Here's how the part is built. I have some questions about the finished solid (model axes, mm). Face numbers are marked on the shaded views. Give positions to 0.01 mm unless a question says otherwise; leave off trailing zeros. Order: outer loops, then holes, each group sorted by start corner. A loop starts at its lowest first (then second) coordinate and runs counter-clockwise, first axis right, second up. Notation, with made-up numbers: (-27, 70) - (-13, 70) arc R20 ccw to (-13, 81) - close; hole circle Ø1 at (72, 51.5). An arc over 180 degrees is marked (long way). One line per question, with ' | ' between items.
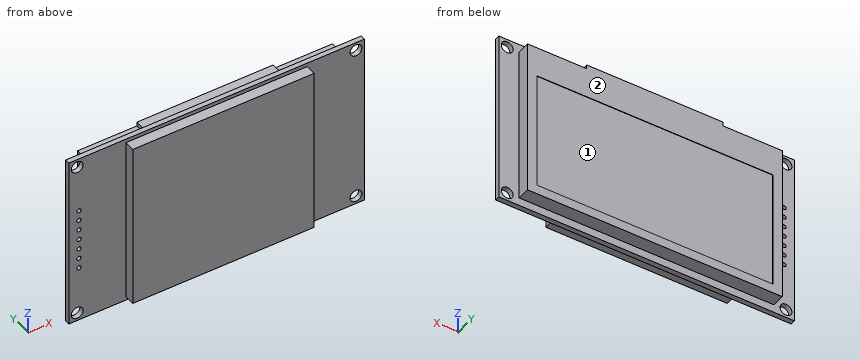
from build123d import *

# Parameters (mm, degrees)
SKETCH1_W           = 72.5
SKETCH1_H           = 43
SKETCH1_R           = 1.45
SKETCH1_R_2         = 0.5
BOSS_EXTRUDE1_DEPTH = 1.2
SKETCH2_W           = 44.5
SKETCH2_H           = 41.146019014
BOSS_EXTRUDE2_DEPTH = 2.6
BOSS_EXTRUDE3_DEPTH = 3.13
SKETCH4_W           = 57.9
SKETCH4_H           = 29.2
CUT_EXTRUDE1_DEPTH  = 0.1


with BuildPart() as part:
    # Sketch1 → Boss-Extrude1 (new body)
    with BuildSketch(Plane(origin=(0, 0, 0), x_dir=(1, 0, 0), z_dir=(0, 1, 0))):
        Rectangle(SKETCH1_W, SKETCH1_H)
        with Locations((-34.2, 19.45)):
            Circle(SKETCH1_R, mode=Mode.SUBTRACT)
        with Locations((-33.75, 7.62)):
            Circle(SKETCH1_R_2, mode=Mode.SUBTRACT)
        with Locations((-33.75, 5.08)):
            Circle(SKETCH1_R_2, mode=Mode.SUBTRACT)
        with Locations((-33.75, 2.54)):
            Circle(SKETCH1_R_2, mode=Mode.SUBTRACT)
        with Locations((-33.75, 0)):
            Circle(SKETCH1_R_2, mode=Mode.SUBTRACT)
        with Locations((-33.75, -2.54)):
            Circle(SKETCH1_R_2, mode=Mode.SUBTRACT)
        with Locations((-33.75, -5.08)):
            Circle(SKETCH1_R_2, mode=Mode.SUBTRACT)
        with Locations((-33.75, -7.62)):
            Circle(SKETCH1_R_2, mode=Mode.SUBTRACT)
        with Locations((-34.2, -19.45)):
            Circle(SKETCH1_R, mode=Mode.SUBTRACT)
        with Locations((34.2, 19.45)):
            Circle(SKETCH1_R, mode=Mode.SUBTRACT)
        with Locations((34.2, -19.45)):
            Circle(SKETCH1_R, mode=Mode.SUBTRACT)
    extrude(amount=-BOSS_EXTRUDE1_DEPTH)

    # Sketch2 → Boss-Extrude2 (add)
    with BuildSketch(Plane.XZ.offset(1.2)):
        Rectangle(SKETCH2_W, SKETCH2_H)
    extrude(amount=BOSS_EXTRUDE2_DEPTH)

    # Sketch3 → Boss-Extrude3 (add)
    with BuildSketch(Plane(origin=(0, 0, 0), x_dir=(1, 0, 0), z_dir=(0, 1, 0))):
        Polygon((-16.75, -19.5), (-16.75, -20.5), (16.75, -20.5), (16.75, -19.5), (31.25, -19.5), (31.25, 19.5), (-31.25, 19.5), (-31.25, -19.5), align=None)
    extrude(amount=BOSS_EXTRUDE3_DEPTH)

    # Sketch4 → Cut-Extrude1 (cut)
    with BuildSketch(Plane(origin=(0, 3.13, 0), x_dir=(1, 0, 0), z_dir=(0, 1, 0))):
        with Locations((0, 2.6)):
            Rectangle(SKETCH4_W, SKETCH4_H)
    extrude(amount=-CUT_EXTRUDE1_DEPTH, mode=Mode.SUBTRACT)


solid = part.part
1) I want a section at C-C (z = 17). List the corners of the cut face in (x, y) for me.
Model answer:
outline: (-36.25, -1.2) - (-22.25, -1.2) - (-22.25, -3.8) - (22.25, -3.8) - (22.25, -1.2) - (36.25, -1.2) - (36.25, 0) - (31.25, 0) - (31.25, 3.13) - (-31.25, 3.13) - (-31.25, 0) - (-36.25, 0) - close
2) Thinking about a two-plate mould opening in X: for the marked faces 1 and 2, which applies, +X half, -X half, draft (parallel to the pull), parting line (faces both ways), or undercut?
Model answer:
face 1: undercut | face 2: draft
3) I want a section at A-A (x = 23). List the corners of the cut face in (y, z) for me.
Model answer:
outline: (-1.2, -21.5) - (0, -21.5) - (0, -19.5) - (3.13, -19.5) - (3.13, -17.2) - (3.03, -17.2) - (3.03, 12) - (3.13, 12) - (3.13, 19.5) - (0, 19.5) - (0, 21.5) - (-1.2, 21.5) - close
4) Please list where these lines run through material, in increasing order: L1, parallel to X at y = -0.8, z = 19.45; L2, parallel to Z at x = 34.2, y = -0.9; L3, parallel to X at y = -0.85, z = -5.08.
Model answer:
L1: x = -36.25 to -35.65, -32.75 to 32.75, 35.65 to 36.25 | L2: z = -21.5 to -20.9, -18 to 18, 20.9 to 21.5 | L3: x = -36.25 to -34.25, -33.25 to 36.25
5) I want a section at D-D (x = -16). List the corners of the cut face in (y, z) for me.
Model answer:
outline: (-3.8, -20.57) - (-1.2, -20.57) - (-1.2, -21.5) - (0, -21.5) - (0, -19.5) - (3.13, -19.5) - (3.13, -17.2) - (3.03, -17.2) - (3.03, 12) - (3.13, 12) - (3.13, 20.5) - (0, 20.5) - (0, 21.5) - (-1.2, 21.5) - (-1.2, 20.57) - (-3.8, 20.57) - close
6) I want a section at B-B (y = 1). List the corners of the cut face in (x, z) for me.
Model answer:
outline: (-31.25, -19.5) - (31.25, -19.5) - (31.25, 19.5) - (16.75, 19.5) - (16.75, 20.5) - (-16.75, 20.5) - (-16.75, 19.5) - (-31.25, 19.5) - close
7) I'm going to push flat-ended pins straight in: P1, Ø1.6, axis at x = -14.5, y = 2, coming from the -Z side; P2, Ø4.5, axis at x = 34.2, z = -19.45, coming from the +Y side; P3, Ø0.9, axis at y = 1, z = 1.5, coming from the +X side. Where does each tip first touch, or does it pass through?
Model answer:
P1: stops at z = -19.5 | P2: stops at y = 0 | P3: stops at x = 31.25
